```python
from build123d import *

# Parameters (mm, degrees)
F1_DEPTH = 5


with BuildPart() as f1:
    # F0 (on Top) → F1 (new body)
    with BuildSketch(Plane.XY):
        with BuildLine():
            ThreePointArc((0, 79.5), (-56.2149891043, -56.2149891043), (79.5, 0))
            ThreePointArc((79.5, 0), (56.2149891043, 56.2149891043), (0, 79.5))
        make_face()
        with BuildLine():
            ThreePointArc((-64.5188925819, 37.25), (-37.25, 64.5188925819), (0, 74.5))
            ThreePointArc((0, 74.5), (2.5014103755, 74.4579945079), (5, 74.3320253996))
            ThreePointArc((5, 74.3320253996), (19.2820188601, 71.9614740585), (32.8358856809, 66.8734223108))
            ThreePointArc((32.8358856809, 66.8734223108), (35.0627123235, 65.7332199464), (37.25, 64.5188925819))
            ThreePointArc((37.25, 64.5188925819), (64.5188925819, 37.25), (74.5, 0))
            ThreePointArc((74.5, 0), (74.4579945079, -2.5014103755), (74.3320253996, -5))
            ThreePointArc((74.3320253996, -5), (71.9614740585, -19.2820188601), (66.8734223108, -32.8358856809))
            ThreePointArc((66.8734223108, -32.8358856809), (65.7332199464, -35.0627123235), (64.5188925819, -37.25))
            ThreePointArc((64.5188925819, -37.25), (37.25, -64.5188925819), (0, -74.5))
            ThreePointArc((0, -74.5), (-2.5014103755, -74.4579945079), (-5, -74.3320253996))
            ThreePointArc((-5, -74.3320253996), (-19.2820188601, -71.9614740585), (-32.8358856809, -66.8734223108))
            ThreePointArc((-32.8358856809, -66.8734223108), (-35.0627123235, -65.7332199464), (-37.25, -64.5188925819))
            ThreePointArc((-37.25, -64.5188925819), (-64.5188925819, -37.25), (-74.5, 0))
            ThreePointArc((-74.5, 0), (-74.4579945079, 2.5014103755), (-74.3320253996, 5))
            ThreePointArc((-74.3320253996, 5), (-71.9614740585, 19.2820188601), (-66.8734223108, 32.8358856809))
            ThreePointArc((-66.8734223108, 32.8358856809), (-65.7332199464, 35.0627123235), (-64.5188925819, 37.25))
        make_face(mode=Mode.SUBTRACT)
        with BuildLine():
            Line((-8.6602540378, 5), (-64.5188925819, 37.25))
            ThreePointArc((-64.5188925819, 37.25), (-65.7332199464, 35.0627123235), (-66.8734223108, 32.8358856809))
            Line((-66.8734223108, 32.8358856809), (-18.6602540378, 5))
            Line((-18.6602540378, 5), (-74.3320253996, 5))
            ThreePointArc((-74.3320253996, 5), (-74.4579945079, 2.5014103755), (-74.5, 0))
            Line((-74.5, 0), (-10, 0))
            ThreePointArc((-10, 0), (-9.6592582629, 2.588190451), (-8.6602540378, 5))
        make_face()
        with BuildLine():
            Line((74.5, 0), (10, 0))
            ThreePointArc((10, 0), (9.6592582629, -2.588190451), (8.6602540378, -5))
            Line((8.6602540378, -5), (64.5188925819, -37.25))
            ThreePointArc((64.5188925819, -37.25), (65.7332199464, -35.0627123235), (66.8734223108, -32.8358856809))
            Line((66.8734223108, -32.8358856809), (18.6602540378, -5))
            Line((18.6602540378, -5), (74.3320253996, -5))
            ThreePointArc((74.3320253996, -5), (74.4579945079, -2.5014103755), (74.5, 0))
        make_face()
        with BuildLine():
            ThreePointArc((0, -10), (-2.588190451, -9.6592582629), (-5, -8.6602540378))
            Line((-5, -8.6602540378), (-37.25, -64.5188925819))
            ThreePointArc((-37.25, -64.5188925819), (-35.0627123235, -65.7332199464), (-32.8358856809, -66.8734223108))
            Line((-32.8358856809, -66.8734223108), (-5, -18.6602540378))
            Line((-5, -18.6602540378), (-5, -74.3320253996))
            ThreePointArc((-5, -74.3320253996), (-2.5014103755, -74.4579945079), (0, -74.5))
            Line((0, -74.5), (0, -10))
        make_face()
        with BuildLine():
            ThreePointArc((5, 74.3320253996), (2.5014103755, 74.4579945079), (0, 74.5))
            Line((0, 74.5), (0, 10))
            ThreePointArc((0, 10), (2.588190451, 9.6592582629), (5, 8.6602540378))
            Line((5, 8.6602540378), (37.25, 64.5188925819))
            ThreePointArc((37.25, 64.5188925819), (35.0627123235, 65.7332199464), (32.8358856809, 66.8734223108))
            Line((32.8358856809, 66.8734223108), (5, 18.6602540378))
            Line((5, 18.6602540378), (5, 74.3320253996))
        make_face()
        with BuildLine():
            ThreePointArc((8.6602540378, -5), (9.6592582629, -2.588190451), (10, 0))
            Line((10, 0), (2.5, 0))
            ThreePointArc((2.5, 0), (2.4148145657, -0.6470476128), (2.1650635095, -1.25))
            Line((2.1650635095, -1.25), (8.6602540378, -5))
        make_face()
        with BuildLine():
            ThreePointArc((0, -10), (5, -8.6602540378), (8.6602540378, -5))
            Line((8.6602540378, -5), (2.1650635095, -1.25))
            ThreePointArc((2.1650635095, -1.25), (1.8705073194, -1.6586748831), (1.5, -2))
            ThreePointArc((1.5, -2), (0.790569415, -2.3717082451), (0, -2.5))
            Line((0, -2.5), (0, -10))
        make_face()
        with BuildLine():
            ThreePointArc((10, 0), (8.6602540378, 5), (5, 8.6602540378))
            Line((5, 8.6602540378), (1.25, 2.1650635095))
            ThreePointArc((1.25, 2.1650635095), (1.3774746787, 2.0862798253), (1.5, 2))
            ThreePointArc((1.5, 2), (2.2360679775, 1.1180339887), (2.5, 0))
            Line((2.5, 0), (10, 0))
        make_face()
        with BuildLine():
            ThreePointArc((5, 8.6602540378), (2.588190451, 9.6592582629), (0, 10))
            Line((0, 10), (0, 2.5))
            ThreePointArc((0, 2.5), (0.6470476128, 2.4148145657), (1.25, 2.1650635095))
            Line((1.25, 2.1650635095), (5, 8.6602540378))
        make_face()
        with BuildLine():
            Line((0, 2.5), (0, 10))
            ThreePointArc((0, 10), (-5, 8.6602540378), (-8.6602540378, 5))
            Line((-8.6602540378, 5), (-2.1650635095, 1.25))
            ThreePointArc((-2.1650635095, 1.25), (-1.8705073194, 1.6586748831), (-1.5, 2))
            ThreePointArc((-1.5, 2), (-0.790569415, 2.3717082451), (0, 2.5))
        make_face()
        with BuildLine():
            Line((-2.1650635095, 1.25), (-8.6602540378, 5))
            ThreePointArc((-8.6602540378, 5), (-9.6592582629, 2.588190451), (-10, 0))
            Line((-10, 0), (-2.5, 0))
            ThreePointArc((-2.5, 0), (-2.4148145657, 0.6470476128), (-2.1650635095, 1.25))
        make_face()
        with BuildLine():
            Line((-2.5, 0), (-10, 0))
            ThreePointArc((-10, 0), (-8.6602540378, -5), (-5, -8.6602540378))
            Line((-5, -8.6602540378), (-1.25, -2.1650635095))
            ThreePointArc((-1.25, -2.1650635095), (-1.3774746787, -2.0862798253), (-1.5, -2))
            ThreePointArc((-1.5, -2), (-2.2360679775, -1.1180339887), (-2.5, 0))
        make_face()
        with BuildLine():
            Line((-1.25, -2.1650635095), (-5, -8.6602540378))
            ThreePointArc((-5, -8.6602540378), (-2.588190451, -9.6592582629), (0, -10))
            Line((0, -10), (0, -2.5))
            ThreePointArc((0, -2.5), (-0.6470476128, -2.4148145657), (-1.25, -2.1650635095))
        make_face()
        with BuildLine():
            ThreePointArc((2.1650635095, -1.25), (2.4148145657, -0.6470476128), (2.5, 0))
            Line((2.5, 0), (1.5, 0))
            Line((1.5, 0), (1.5, -0.8660254038))
            Line((1.5, -0.8660254038), (2.1650635095, -1.25))
        make_face()
        with BuildLine():
            Line((1.5, 0), (2.5, 0))
            ThreePointArc((2.5, 0), (2.2360679775, 1.1180339887), (1.5, 2))
            Line((1.5, 2), (1.5, 0))
        make_face()
        with BuildLine():
            Line((2.1650635095, -1.25), (1.5, -0.8660254038))
            Line((1.5, -0.8660254038), (1.5, -2))
            ThreePointArc((1.5, -2), (1.8705073194, -1.6586748831), (2.1650635095, -1.25))
        make_face()
        with BuildLine():
            Line((-1.5, 0), (-2.5, 0))
            ThreePointArc((-2.5, 0), (-2.2360679775, -1.1180339887), (-1.5, -2))
            Line((-1.5, -2), (-1.5, 0))
        make_face()
        with BuildLine():
            Line((-1.5, 0.8660254038), (-2.1650635095, 1.25))
            ThreePointArc((-2.1650635095, 1.25), (-2.4148145657, 0.6470476128), (-2.5, 0))
            Line((-2.5, 0), (-1.5, 0))
            Line((-1.5, 0), (-1.5, 0.8660254038))
        make_face()
        with BuildLine():
            ThreePointArc((-1.5, 2), (-1.8705073194, 1.6586748831), (-2.1650635095, 1.25))
            Line((-2.1650635095, 1.25), (-1.5, 0.8660254038))
            Line((-1.5, 0.8660254038), (-1.5, 2))
        make_face()
    extrude(amount=F1_DEPTH)


solid = f1.part
```
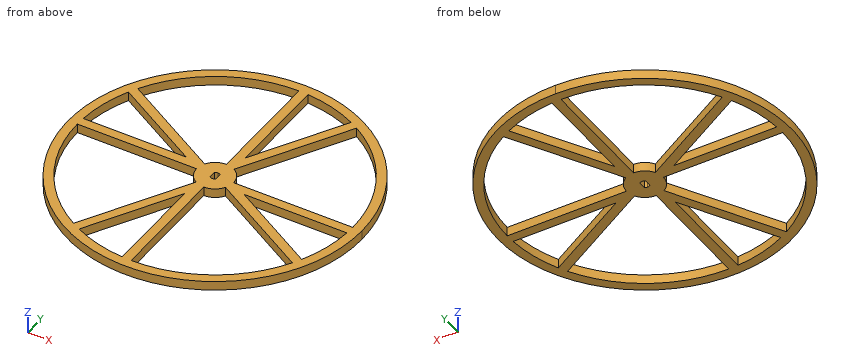
Verification items for the finished model (mm, model axes). Round coordinates to 2 decimals unless told otherwise and drop trailing zeros. Loops run counter-clockwise (first coordinate to the right, second up) from the corner with the lowest first, then second, coordinate; pieces in that order, holes last. Notation, with made-up numbers: (77.25, -32.5) -> (106.25, -32.5) arc R16 ccw to (106.25, -9.5) -> close; hole circle Ø11 at (-24, 80). An arc over 180 degrees is marked (long way). Answer as a JSON object with one key per item and string values.
Q1. Section check C-C (x = -47). Record the boundary of the cut face in (y, z), then the cut area to 3 significant figures.
Data:
{"outline": "(-64.12, 0) -> (-57.8, 0) -> (-57.8, 5) -> (-64.12, 5) -> close; (0, 0) -> (5, 0) -> (5, 5) -> (0, 5) -> close; (21.36, 0) -> (27.14, 0) -> (27.14, 5) -> (21.36, 5) -> close; (57.8, 0) -> (64.12, 0) -> (64.12, 5) -> (57.8, 5) -> close", "area": "117 mm2"}
Q2. Section check B-B (z = 2.4). State how many separate pieces and enclosed holes the cut face has, then the cut area to 3 significant figures.
Data:
{"separate pieces": "1", "enclosed holes": "9", "area": "5,220 mm2"}
Q3. Section check A-A (x = -28.5). Record the boundary of the cut face in (y, z).
Data:
{"outline": "(-74.22, 0) -> (-68.83, 0) -> (-68.83, 5) -> (-74.22, 5) -> close; (-59.36, 0) -> (-49.36, 0) -> (-49.36, 5) -> (-59.36, 5) -> close; (0, 0) -> (5, 0) -> (5, 5) -> (0, 5) -> close; (10.68, 0) -> (16.45, 0) -> (16.45, 5) -> (10.68, 5) -> close; (68.83, 0) -> (74.22, 0) -> (74.22, 5) -> (68.83, 5) -> close"}
Q4. Go/stop test with flat-tipped pins: P1, Ø1.5, axis at x = -36, z = 3, coming from the -Y side; P2, Ø1.5, axis at y = 32, z = 3.5, coming from the -X side; P3, Ø2, axis at y = -53, z = 3.5, coming from the +X side. Record where each tip stops, or that it passes through.
Data:
{"P1": "stops at y = -71.26", "P2": "stops at x = -73.1", "P3": "stops at x = 60.14"}
Q5. Scan lines: line 1 (Y direction, x = -18, z = 0.5); line 2 (X direction, y = -41.5, z = 1.05); line 3 (Y direction, x = -26, z = 2.65). Record each from-to range of solid material in increasing order. Write a range as from..to.
Data:
{"line 1": "y = -77.44..-72.29, -41.18..-31.18, 0..10.39, 72.29..77.44", "line 2": "x = -67.81..-61.87, -23.96..-18.19, -5..0, 61.87..67.81", "line 3": "y = -75.13..-69.82, -55.03..-45.03, 0..5, 9.24..15.01, 69.82..75.13"}
Q6. Section check D-D (x = 31). Record the boundary of the cut face in (y, z).
Data:
{"outline": "(-73.21, 0) -> (-67.74, 0) -> (-67.74, 5) -> (-73.21, 5) -> close; (-17.9, 0) -> (-12.12, 0) -> (-12.12, 5) -> (-17.9, 5) -> close; (-5, 0) -> (0, 0) -> (0, 5) -> (-5, 5) -> close; (53.69, 0) -> (63.69, 0) -> (63.69, 5) -> (53.69, 5) -> close; (67.74, 0) -> (73.21, 0) -> (73.21, 5) -> (67.74, 5) -> close"}
